from build123d import *

# Parameters (mm, degrees)
SKETCH2_W           = 28.58
SKETCH2_H           = 39.94
BOSS_EXTRUDE1_DEPTH = 11.7
FILLET1_R           = 15.4
BOSS_EXTRUDE2_DEPTH = 11.7
SKETCH3_R           = 1.5
CUT_EXTRUDE1_DEPTH  = 11.7
SKETCH6_R           = 3
CUT_EXTRUDE2_DEPTH  = 11.7


with BuildPart() as part:
    # Sketch2 → Boss-Extrude1 (new body)
    with BuildSketch(Plane(origin=(0, 0, 0), x_dir=(0, 0, -1), z_dir=(1, 0, 0))):
        with Locations((-28.077336683, 0.926432161)):
            Rectangle(SKETCH2_W, SKETCH2_H)
    extrude(amount=BOSS_EXTRUDE1_DEPTH)

    # Fillet1
    # the kernel refuses this fillet: 15.4 mm, written as the material it takes off along each edge
    with BuildSketch(Plane(origin=(-38.5, 20.896432161, 13.787336683), x_dir=(0, -1, 0), z_dir=(1, 0, 0))) as fillet1_piece_1:
        with BuildLine():
            CenterArc((FILLET1_R, -FILLET1_R), FILLET1_R, 90, 90)
            Line((0, -FILLET1_R), (0, 0))
            Line((0, 0), (FILLET1_R, 0))
        make_face()
    extrude(amount=88.7, mode=Mode.SUBTRACT)
    with BuildSketch(Plane(origin=(-38.5, 20.896432161, 42.367336683), x_dir=(0, -1, 0), z_dir=(1, 0, 0))) as fillet1_piece_2:
        with BuildLine():
            CenterArc((FILLET1_R, FILLET1_R), FILLET1_R, 180, 90)
            Line((0, FILLET1_R), (0, 0))
            Line((0, 0), (FILLET1_R, 0))
        make_face()
    extrude(amount=88.7, mode=Mode.SUBTRACT)

    # Sketch5 → Boss-Extrude2 (add)
    with BuildSketch(Plane(origin=(11.7, 0, 0), x_dir=(0, 0, -1), z_dir=(1, 0, 0))):
        Polygon((-42.141577226, 8.123678622), (-47.367336683, 6.723440596), (-47.367336683, 3.723440596), (-42.367336683, 3.723440596), align=None)
        Polygon((-13.787336683, 3.723440596), (-8.787336683, 3.723440596), (-8.787336683, 6.723440596), (-14.013096141, 8.123678622), align=None)
    extrude(amount=-BOSS_EXTRUDE2_DEPTH)

    # Sketch3 → Cut-Extrude1 (cut)
    with BuildSketch(Plane(origin=(11.7, 0, 0), x_dir=(0, 0, -1), z_dir=(1, 0, 0))):
        with Locations((-44.297336683, 5.526376822)):
            Circle(SKETCH3_R)
        with Locations((-11.857336683, 5.526376822)):
            Circle(SKETCH3_R)
    extrude(amount=-CUT_EXTRUDE1_DEPTH, mode=Mode.SUBTRACT)

    # Sketch6 → Cut-Extrude2 (cut)
    with BuildSketch(Plane(origin=(11.7, 0, 0), x_dir=(0, 0, -1), z_dir=(1, 0, 0))):
        with Locations((-28.077336683, 5.526376822)):
            Circle(SKETCH6_R)
    extrude(amount=-CUT_EXTRUDE2_DEPTH, mode=Mode.SUBTRACT)


solid = part.part
The listing builds one solid part. Answer for the finished solid, in the listing's coordinates (mm). A direction names the side the tool comes from. Coordinates: 2 decimals unless noted, no trailing zeros. Order: outer loops, then holes, each group sorted by start corner. A loop starts at its lowest first (then second) coordinate and runs counter-clockwise, first axis right, second up.
Q1. Given P1, Ø3, axis at x = 1.5, y = 7, coming from the +Z side; P2, Ø2, axis at x = 7.5, y = -15, coming from the -Z side; P3, Ø1.5, axis at x = 3.5, z = 44.5, coming from the -Y side; P4, Ø5, axis at y = 5.53, z = 28.08, coming from the -X side, each flat-ended and moving along its own axis, determine where each tip first touches the part or whether it passes through.
Q2. A cutting plane is placed at A-A, the plane x = 7.5. Write down the section's boundary in (y, z), and give its area (3 significant figures).
Q3. A cutting plane is placed at C-C, the plane y = 2. Write down the section's boundary in (x, z).
Q4. Which of the six approach directions +Z, -Z, +X, -X, +Y, -Y give full straight-line access (tool end or side, diameter ignored) to faces 5 (the face through (6, -8, 13.787)), 6 (the face through (6, 5, 8.787)), 7 (the face through (6, -8, 42.367))?
Q5. A cutting plane is placed at B-B, the plane z = 37. Write down the section's boundary in (x, y).
Q6. For a pull along Z with two mould halves and no side action, classify faces 1 (the face through (5.77, 16.82, 18.75)), 2 (the face through (5.768, 17.008, 37.196)), 3 (the face through (0, 1, 28)), 4 (the face through (5.932, 6.427, 25.216)) as pulls with the +Z half, pulls with the -Z half, needs draft (parallel to the pull), parting line crosses it, or undercut.
Q7. Consider line 1 (Z direction, x = 2.25, y = 6.5); line 2 (Z direction, x = 10.5, y = -15.5); line 3 (Y direction, x = 3.75, z = 44). Determine where each line is inside the solid, lowest interval first.
Answers follow:
1. P1: stops at z = 47.37
1. P2: stops at z = 13.79
1. P3: stops at y = 3.72
1. P4: passes through
2. outline: (-19.04, 13.79) - (3.72, 13.79) - (3.72, 8.79) - (6.72, 8.79) - (8.12, 14.01) arc R15.4 ccw to (20.86, 28.08) arc R15.4 ccw to (8.12, 42.14) - (6.72, 47.37) - (3.72, 47.37) - (3.72, 42.37) - (-19.04, 42.37) - close; hole circle Ø6 at (5.53, 28.08); hole circle Ø3 at (5.53, 11.86); hole circle Ø3 at (5.53, 44.3)
2. area: 1,030 mm2
3. outline: (0, 13.79) - (11.7, 13.79) - (11.7, 42.37) - (0, 42.37) - close
4. face 5: -Z, +X, -X, -Y
4. face 6: -Z, +X, -X, +Y, -Y
4. face 7: +Z, +X, -X, -Y
5. outline: (0, -19.04) - (11.7, -19.04) - (11.7, 17.18) - (0, 17.18) - close
6. face 1: pulls with the -Z half
6. face 2: pulls with the +Z half
6. face 3: needs draft
6. face 4: undercut
7. line 1: z = 8.79 to 10.72, 13 to 25.24, 30.91 to 43.16, 45.44 to 47.37
7. line 2: z = 13.79 to 42.37
7. line 3: y = 3.72 to 4.06, 7 to 7.63
